Here's how the part is built. I have some questions about the finished solid (model axes, mm). A direction names the side the tool comes from. Round coordinates to 2 decimals unless told otherwise and drop trailing zeros. Order: outer loops, then holes, each group sorted by start corner. A loop starts at its lowest first (then second) coordinate and runs counter-clockwise, first axis right, second up.
```python
from build123d import *

# Parameters (mm, degrees)
BOSS_EXTRUDE1_DEPTH = 8
SKETCH2_R           = 4.7625
SKETCH2_R_2         = 3
CUT_EXTRUDE1_DEPTH  = 20
SKETCH3_R           = 4
CUT_EXTRUDE2_DEPTH  = 0.5
SKETCH4_R           = 2.5
CUT_EXTRUDE3_DEPTH  = 20


with BuildPart() as part:
    # Sketch1 → Boss-Extrude1 (new body)
    with BuildSketch(Plane.XY):
        with BuildLine():
            Line((0, -8), (160, -8))
            Line((160, -8), (160, 8))
            Line((160, 8), (0, 8))
            ThreePointArc((0, 8), (-8, 0), (0, -8))
        make_face()
    extrude(amount=BOSS_EXTRUDE1_DEPTH)

    # Sketch2 → Cut-Extrude1 (cut, symmetric)
    with BuildSketch(Plane.XY):
        Circle(SKETCH2_R)
        with Locations((150, 0)):
            Circle(SKETCH2_R_2)
    extrude(amount=CUT_EXTRUDE1_DEPTH, both=True, mode=Mode.SUBTRACT)

    # Sketch3 → Cut-Extrude2 (cut, symmetric)
    with BuildSketch(Plane.XY):
        with Locations((30, 0)):
            Circle(SKETCH3_R)
    extrude(amount=CUT_EXTRUDE2_DEPTH, both=True, mode=Mode.SUBTRACT)

    # Sketch4 → Cut-Extrude3 (cut, symmetric)
    with BuildSketch(Plane(origin=(0, 0, 0), x_dir=(1, 0, 0), z_dir=(0, 1, 0))):
        with Locations(Location((0, -4, 0), (0, 0, 270))):
            Circle(SKETCH4_R)
    extrude(amount=CUT_EXTRUDE3_DEPTH, both=True, mode=Mode.SUBTRACT)


solid = part.part
```
1) If we section it at D-D (x = 30): Write out the boundary of the cut face in (y, z), plus the area to 3 significant figures.
2) I need wall thicknesses on line 1 (Z direction, x = 0, y = -6.3); line 2 (X direction, y = 2.5, z = 7.75); line 3 (X direction, y = 1, z = 6.25). Which ranges of each line are inside material? Lowest first, please.
3) For faces 1 (the flat face through (75, 0, 8)), 2 (the cylindrical face through (26.8, -2.4, 0.3)), which set-ups out of +Z, -Z, +X, -X, +Y, -Y let a thin tool reach every point of the face, with its end or its side?
4) I'm going to push flat-ended pins straight in: pin 1 (2 mm diameter, centred on y = 3, z = 6.5, fed in from -X); pin 2 (5.5 mm diameter, centred on x = 150, y = 0, fed in from -Z). Where does each tip first touch, or does it pass through?
5) If we section it at A-A (x = 150): Write out the boundary of the cut face in (y, z), plus the area to 3 significant figures.
6) If we section it at B-B (z = 3): Write out the boundary of the cut face in (x, y) (1 decimal), plus the area to 3 significant figures.
7) If we section it at C-C (y = 1.5): Write out the boundary of the cut face in (x, z).
8) We'd pull the mould along Y, two halves only. Please class faces 3 (the cylindrical face through (-8, 0, 4)), 4 (the cylindrical face through (2.48, -6, 3.67)), 5 (the flat face through (30, 0, 0.5)): +Y half, -Y half, draft (parallel to the pull), parting line (faces both ways), or undercut.
Solutions:
1. outline: (-8, 0) - (-4, 0) - (-4, 0.5) - (4, 0.5) - (4, 0) - (8, 0) - (8, 8) - (-8, 8) - close
1. area: 124 mm2
2. line 1: z = 0 to 1.5, 6.5 to 8
2. line 2: x = -7.6 to -4.05, 4.05 to 148.34, 151.66 to 160
2. line 3: x = -7.94 to -4.66, 4.66 to 147.17, 152.83 to 160
3. face 1: +Z, +X, -X, +Y, -Y
3. face 2: -Z
4. pin 1: stops at x = -7.75
4. pin 2: passes through
5. outline: (-8, 0) - (-3, 0) - (-3, 8) - (-8, 8) - close; (3, 0) - (8, 0) - (8, 8) - (3, 8) - close
5. area: 80.0 mm2
6. outline: (-2.3, -7.7) - (-2.3, -4.2) arc R4.8 cw to (-2.3, 4.2) - (-2.3, 7.7) arc R8 ccw to start; (2.3, -8) - (160, -8) - (160, 8) - (2.3, 8) - (2.3, 4.2) arc R4.8 cw to (2.3, -4.2) - close; hole circle Ø6 at (150, 0)
6. area: 2,530 mm2
7. outline: (-7.86, 0) - (-4.52, 0) - (-4.52, 8) - (-7.86, 8) - close; (4.52, 0) - (26.29, 0) - (26.29, 0.5) - (33.71, 0.5) - (33.71, 0) - (147.4, 0) - (147.4, 8) - (4.52, 8) - close; (152.6, 0) - (160, 0) - (160, 8) - (152.6, 8) - close
8. face 3: parting line
8. face 4: draft
8. face 5: undercut
